```python
from build123d import *

# Parameters (mm, degrees)
SKETCH1_W           = 40
SKETCH1_H           = 40
BOSS_EXTRUDE1_DEPTH = 4
FILLET2_R           = 2
SHELL1_START        = 2
SHELL1_OUTLINE_W    = 2
SHELL1_OUTLINE_H    = 36
SHELL1_DEPTH        = 36
SKETCH2_W           = 26
SKETCH2_H           = 16
CUT_EXTRUDE1_DEPTH  = 4


# Read off the part's stored shape, not the designer's step: Shell1
with BuildPart() as part:
    # Sketch1 → Boss-Extrude1 (new body)
    with BuildSketch(Plane(origin=(0, 0, 0), x_dir=(1, 0, 0), z_dir=(0, 1, 0))):
        with Locations((20, 20)):
            Rectangle(SKETCH1_W, SKETCH1_H)
    extrude(amount=BOSS_EXTRUDE1_DEPTH)

    # Fillet2
    fillet2_edges = [part.edges().sort_by_distance(p)[0] for p in [
        (40, 4, -20),
        (20, 4, -40),
        (0, 4, -20),
        (20, 4, 0),
    ]]
    fillet(fillet2_edges, radius=FILLET2_R)

    # Shell1 outline → Shell1 (cut)
    with BuildSketch(Plane.YZ.offset(SHELL1_START)):
        with Locations((1, -20)):
            Rectangle(SHELL1_OUTLINE_W, SHELL1_OUTLINE_H)
    extrude(amount=SHELL1_DEPTH, mode=Mode.SUBTRACT)

    # Sketch2 → Cut-Extrude1 (cut)
    with BuildSketch(Plane(origin=(0, 4, 0), x_dir=(1, 0, 0), z_dir=(0, 1, 0))):
        with Locations((20, 20)):
            Rectangle(SKETCH2_W, SKETCH2_H)
    extrude(amount=-CUT_EXTRUDE1_DEPTH, mode=Mode.SUBTRACT)


solid = part.part
```
Work out the finished part from the listing and answer in its coordinate system (mm). A direction names the side the tool comes from. Round coordinates to 2 decimals unless told otherwise and drop trailing zeros. Order: outer loops, then holes, each group sorted by start corner. A loop starts at its lowest first (then second) coordinate and runs counter-clockwise, first axis right, second up.
Q1. A tool of negligible diameter and unlimited length cuts with its end or side. For faces 4 (the flat face through (19.7, 2, -28.3)), 5 (the flat face through (0, 1, -20)), 6 (the flat face through (7, 3, -20)), from which of +Z, -Z, +X, -X, +Y, -Y can it reach the whole face along a straight path? Write none if from no direction.
Solution:
face 4: -Y
face 5: +Z, -Z, -X, +Y, -Y
face 6: +Y, -Y
Q2. A cutting plane is placed at C-C, the plane z = -15.5. Determine the outline of the cut face in (x, y).
Solution:
outline: (0, 0) - (2, 0) - (2, 2) - (7, 2) - (7, 4) - (2, 4) arc R2 ccw to (0, 2) - close; (33, 2) - (38, 2) - (38, 0) - (40, 0) - (40, 2) arc R2 ccw to (38, 4) - (33, 4) - close
Q3. Given pin 1 Ø1.6 at (x, y) = (18.5, 3) entering from +Z; pin 2 Ø1 at (y, z) = (3, -16) entering from +X; pin 3 Ø1 at (x, z) = (27, -13) entering from +Y; pin 4 Ø1 at (x, y) = (10, 3.5) entering from +Z, each flat-ended and moving along its own axis, determine where each tip first touches the part or whether it passes through.
Solution:
pin 1: stops at z = -0.01
pin 2: stops at x = 39.94
pin 3: passes through
pin 4: stops at z = -0.27
Q4. A cutting plane is placed at D-D, the plane z = -35. Determine the outline of the cut face in (x, y), then the cut area to 3 significant figures.
Solution:
outline: (0, 0) - (2, 0) - (2, 2) - (38, 2) - (38, 0) - (40, 0) - (40, 2) arc R2 ccw to (38, 4) - (2, 4) arc R2 ccw to (0, 2) - close
area: 86.3 mm2
Q5. A cutting plane is placed at B-B, the plane y = 1.3. Determine the outline of the cut face in (x, z), then the cut area to 3 significant figures.
Solution:
outline: (0, -40) - (40, -40) - (40, 0) - (0, 0) - close; hole (2, -38) - (38, -38) - (38, -2) - (2, -2) - close
area: 304 mm2
Q6. The mould has two halves that part along X. Classify faces 1 (the flat face through (20, 1, -2)), 2 (the cylindrical face through (20.28, 3.4, -0.57)), 3 (the cylindrical face through (0.57, 3.4, -20.28)): pulls with the +X half, pulls with the -X half, needs draft (parallel to the pull), parting line crosses it, or undercut.
Solution:
face 1: undercut
face 2: needs draft
face 3: pulls with the -X half
Q7. Find the intervals of material crossed by line 1 along X through (y, z) = (1.15, -12); line 2 along Z through (x, y) = (8.5, 1.8); line 3 along Y through (x, z) = (37, -4), in increasing order.
Solution:
line 1: x = 0 to 2, 38 to 40
line 2: z = -40 to -38, -2 to 0
line 3: y = 2 to 4
Q8. A cutting plane is placed at A-A, the plane x = 11. Determine the outline of the cut face in (y, z), then the cut area to 3 significant figures.
Solution:
outline: (0, -40) - (2, -40) arc R2 ccw to (4, -38) - (4, -28) - (2, -28) - (2, -38) - (0, -38) - close; (0, -2) - (2, -2) - (2, -12) - (4, -12) - (4, -2) arc R2 ccw to (2, 0) - (0, 0) - close
area: 54.3 mm2
